Geometry check sheet. Reference: the model listing, model coordinates, mm. Face numbers are marked on the shaded views. A direction names the side the tool comes from. Round coordinates to 2 decimals unless told otherwise and drop trailing zeros. Write each loop counter-clockwise with the first axis right and the second up, starting at its lowest first coordinate (ties: lowest second). Pieces come first, ordered by that corner, then holes. Notation, with made-up numbers: (72.25, 22) - (127.25, 22) arc R6 cw to (127.25, 26) - close; hole circle Ø8 at (32, -13). An arc over 180 degrees is marked (long way). Return JSON: item names as keys, results as strings.
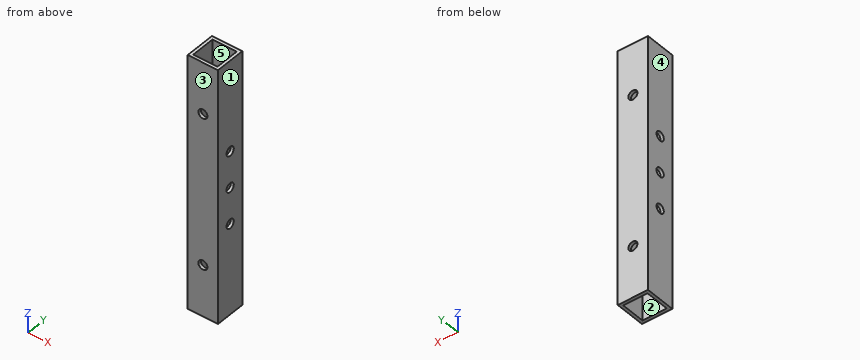
```python
from build123d import *

# Parameters (mm, degrees)
SKETCH_1_W          = 10
SKETCH_1_H          = 10
SKETCH_1_W_2        = 8
SKETCH_1_H_2        = 8
EXTRUDE_1_DEPTH     = 84
SKETCH_2_R          = 1.5
CUT_EXTRUDE_1_DEPTH = 11
SKETCH_3_R          = 1.5
CUT_EXTRUDE_2_DEPTH = 11


with BuildPart() as part:
    # 草图1 → 拉伸-薄壁1 (new body)
    with BuildSketch(Plane.XY):
        Rectangle(SKETCH_1_W, SKETCH_1_H)
        Rectangle(SKETCH_1_W_2, SKETCH_1_H_2, mode=Mode.SUBTRACT)
    extrude(amount=EXTRUDE_1_DEPTH)

    # 草图2 → 切除-拉伸1 (cut, through all)
    with BuildSketch(Plane(origin=(5, 0, 0), x_dir=(0, 0, -1), z_dir=(1, 0, 0))):
        with Locations((-54, 0)):
            Circle(SKETCH_2_R)
        with Locations((-30, 0)):
            Circle(SKETCH_2_R)
        with Locations((-42, 0)):
            Circle(SKETCH_2_R)
    extrude(amount=-CUT_EXTRUDE_1_DEPTH, mode=Mode.SUBTRACT)

    # 草图3 → 切除-拉伸2 (cut, through all)
    with BuildSketch(Plane.XZ.offset(5)):
        with Locations((0, 17)):
            Circle(SKETCH_3_R)
        with Locations((0, 67)):
            Circle(SKETCH_3_R)
    extrude(amount=-CUT_EXTRUDE_2_DEPTH, mode=Mode.SUBTRACT)


solid = part.part
```
(1) Section check B-B, the plane z = 37.5. Enter the section's corners in (x, y).
Response values:
{"outline": "(-5, -5) - (5, -5) - (5, 5) - (-5, 5) - close; hole (-4, -4) - (4, -4) - (4, 4) - (-4, 4) - close"}
(2) Release check for a two-part mould opening along X. For the marked faces 3, 4 and 5 record: pulls with the +X half, pulls with the -X half, needs draft (parallel to the pull), parting line crosses it, or undercut.
Response values:
{"face 3": "needs draft", "face 4": "pulls with the -X half", "face 5": "undercut"}
(3) Section check C-C, the plane z = 54. Enter the section's corners in (x, y).
Response values:
{"outline": "(-5, -5) - (5, -5) - (5, -1.5) - (4, -1.5) - (4, -4) - (-4, -4) - (-4, -1.5) - (-5, -1.5) - close; (-5, 1.5) - (-4, 1.5) - (-4, 4) - (4, 4) - (4, 1.5) - (5, 1.5) - (5, 5) - (-5, 5) - close"}
(4) Access from +Z, -Z, +X, -X, +Y, -Y to the whole of each face (thin tool, end or side, straight path). Record for the marked faces 1 and 2.
Response values:
{"face 1": "+Z, -Z, +X, +Y, -Y", "face 2": "+Z, -Z"}
(5) Gauge pin test, flat end, axial feed: pin 1 (2.5 mm diameter, centred on y = 0, z = 42, fed in from +X). Record the tip position at first contact, or that the pin passes through.
Response values:
{"pin 1": "passes through"}
(6) Section check A-A, the plane x = 2.5. Enter the section's corners in (y, z).
Response values:
{"outline": "(-5, 0) - (-4, 0) - (-4, 84) - (-5, 84) - close; (4, 0) - (5, 0) - (5, 84) - (4, 84) - close"}
(7) Material ranges on line 1 along Z through (x, y) = (0, 4.4); line 2 along X through (y, z) = (-2, 32.5), recorded low to high. Write a range as [from, to].
Response values:
{"line 1": "z = [0, 15.5], [18.5, 65.5], [68.5, 84]", "line 2": "x = [-5, -4], [4, 5]"}
